Geometry: see drawing. Coordinates: mm, zero at the bounding-box minimum. Give positions to 0.01 mm unless a question says otherwise; leave off trailing zeros. Write each loop counter-clockwise with the first axis right and the second up, starting at its lowest first coordinate (ties: lowest second). Pieces come first, ordered by that corner, then holes. Notation, with made-up numbers: (52, -31) -> (74, -31) arc R22 ccw to (74, 2) -> close; hole circle Ø6 at (70.25, 54). An arc over 180 degrees is marked (long way). Answer as a JSON object with one key per item and string values. Group by question number.
Item 1: First-contact query: pin 1 Ø2 at (x, z) = (7.5, 35) entering from +Y; pin 2 Ø4 at (x, y) = (18, 6.5) entering from -Z; pin 3 Ø1.5 at (x, y) = (52.5, 6) entering from +Z; pin 4 Ø1 at (y, z) = (7, 32.5) entering from -X. Flat tips, straight axial feed; report the tip coordinate or a pass-through.
Item 2: Ray query, probe 1 along X at (y, z) = (7.5, 9.5); probe 2 along Y at (x, z) = (14, 4); probe 3 along X at (y, z) = (4.75, 8.5). Return the intervals inside material, ascending. Write a range as from..to.
Item 3: Pull-direction query (Z, two-part tool) for the marked faces 1, 2 and 3; classes: pulls with the +Z half, pulls with the -Z half, needs draft (parallel to the pull), parting line crosses it, or undercut.
Item 4: Section query C-C on z = 10.5. Return the cut outline in (x, y), plus the area to 3 significant figures.
Item 5: Section query A-A on y = 6. Return the cut outline in (x, z), plus the area to 3 significant figures.
Item 6: Section query B-B on x = 52.5. Return the cut outline in (y, z), plus the area to 3 significant figures.
Item 7: Section query D-D on x = 43.5. Return the cut outline in (y, z), plus the area to 3 significant figures.
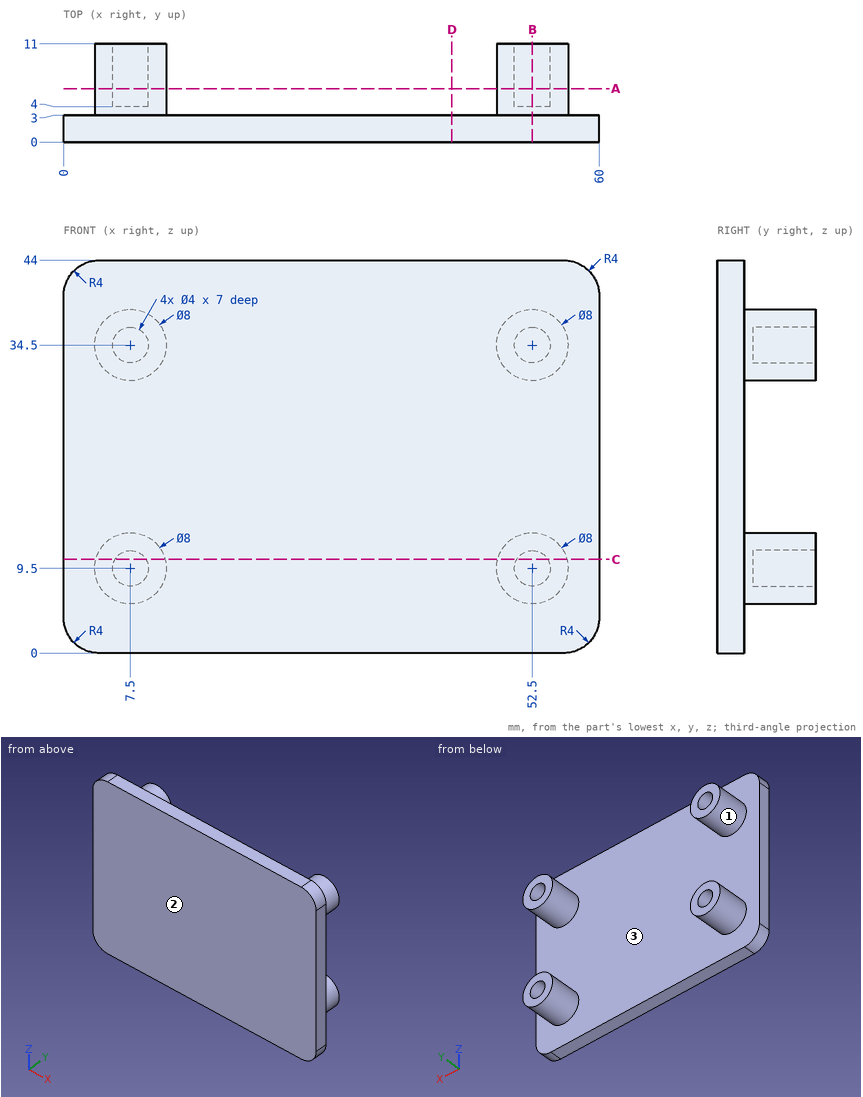
Worked answers:
{
 "1": {"pin 1": "y = 4", "pin 2": "through", "pin 3": "z = 38.5", "pin 4": "x = 3.79"},
 "2": {"probe 1": "3.5..5.5, 9.5..11.5, 48.5..50.5, 54.5..56.5", "probe 2": "0..3", "probe 3": "3.63..5.77, 9.23..11.37, 48.63..50.77, 54.23..56.37"},
 "3": {"face 1": "undercut", "face 2": "needs draft", "face 3": "undercut"},
 "4": {"outline": "(0, 0) -> (60, 0) -> (60, 3) -> (56.37, 3) -> (56.37, 11) -> (54.23, 11) -> (54.23, 4) -> (50.77, 4) -> (50.77, 11) -> (48.63, 11) -> (48.63, 3) -> (11.37, 3) -> (11.37, 11) -> (9.23, 11) -> (9.23, 4) -> (5.77, 4) -> (5.77, 11) -> (3.63, 11) -> (3.63, 3) -> (0, 3) -> close", "area": "255 mm^2"},
 "5": {"outline": "circle Ø8 at (7.5, 9.5); circle Ø8 at (7.5, 34.5); circle Ø8 at (52.5, 9.5); circle Ø8 at (52.5, 34.5); hole circle Ø4 at (7.5, 9.5); hole circle Ø4 at (7.5, 34.5); hole circle Ø4 at (52.5, 9.5); hole circle Ø4 at (52.5, 34.5)", "area": "151 mm^2"},
 "6": {"outline": "(0, 0) -> (3, 0) -> (3, 5.5) -> (11, 5.5) -> (11, 7.5) -> (4, 7.5) -> (4, 11.5) -> (11, 11.5) -> (11, 13.5) -> (3, 13.5) -> (3, 30.5) -> (11, 30.5) -> (11, 32.5) -> (4, 32.5) -> (4, 36.5) -> (11, 36.5) -> (11, 38.5) -> (3, 38.5) -> (3, 44) -> (0, 44) -> close", "area": "204 mm^2"},
 "7": {"outline": "(0, 0) -> (3, 0) -> (3, 44) -> (0, 44) -> close", "area": "132 mm^2"}
}
